Check sheet for the modelled part. Datum: model origin and axes. Units: mm. Face numbers are marked on the shaded views. A direction names the side the tool comes from. Round coordinates to 2 decimals unless told otherwise and drop trailing zeros. Put each result on its own line as item: value. Start each with the question number.
Item 1: Draft check along X on the marked faces 4, 5, 6 and 7. Enter one of: pulls with the +X half, pulls with the -X half, needs draft (parallel to the pull), parting line crosses it, or undercut.
Item 2: Tool access check on the marked faces 1, 2 and 3. Record the directions out of +Z, -Z, +X, -X, +Y, -Y that give a thin tool (end or side, any length) a straight path to the whole face; none if there is none.
Item 3: Section check A-A, the plane z = 2.3. Give the number of separate pieces and of enclosed holes in the cut face, and give its area (3 significant figures).
Item 4: Gauge pin test, flat ends, axial feed: pin 1 Ø4 at (x, y) = (0, 11.11) entering from +Z; pin 2 Ø1 at (x, z) = (4, 1) entering from -Y; pin 3 Ø1 at (x, z) = (9, 1.5) entering from +Y. Record the tip position at first contact, or that the pin passes through.
Item 5: Material ranges on line 1 along Y through (x, z) = (0, 2.05); line 2 along X through (y, z) = (-12.5, 0.8); line 3 along X through (y, z) = (-15, 1.4), recorded low to high.
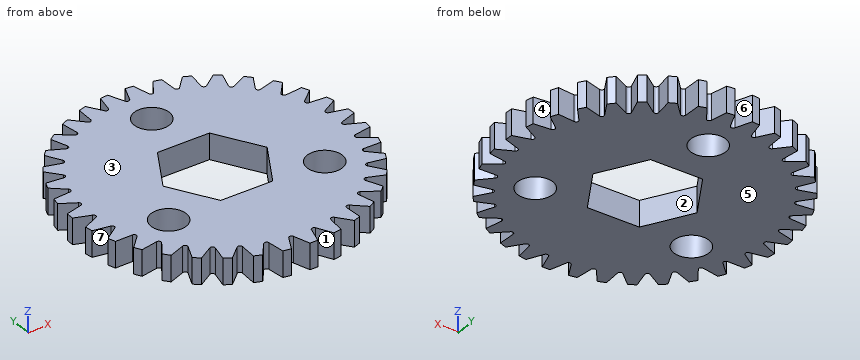
from build123d import *

# Parameters (mm, degrees)
F0_R            = 17.3565013667
F0_R_2          = 2.15265
F1_DEPTH        = 3.175
F3_DEPTH        = 3.175
F3_COPIES_COUNT = 35


# Not quite as in the source:
# - a pattern or mirror of a feature is missing from the dataset's text; its kind, count and spacing are read off the source's solid
# - a feature names something its author has since deleted; it is built from what else it names


with BuildPart() as f1:
    # F0 (on Top) → F1 (new body)
    with BuildSketch(Plane.XY):
        Circle(F0_R)
        with Locations((-9.6237072996, -5.55625)):
            Circle(F0_R_2, mode=Mode.SUBTRACT)
        with Locations((9.6237072996, -5.55625)):
            Circle(F0_R_2, mode=Mode.SUBTRACT)
        Polygon((6.4158048664, 0), (3.2079024332, -5.55625), (-3.2079024332, -5.55625), (-6.4158048664, 0), (-3.2079024332, 5.55625), (3.2079024332, 5.55625), align=None, mode=Mode.SUBTRACT)
        with Locations((0, 11.1125)):
            Circle(F0_R_2, mode=Mode.SUBTRACT)
    extrude(amount=F1_DEPTH)

    # F2 (on face) → F3 (cut, through all)
    with BuildSketch(Plane.XY.offset(3.175)):
        with BuildLine():
            Line((0.275157943, 15.3777549622), (1.0756124971, 17.3231405192))
            ThreePointArc((1.0756124971, 17.3231405192), (0, 17.3565013667), (-1.0756124971, 17.3231405192))
            Line((-1.0756124971, 17.3231405192), (-0.275157943, 15.3777549622))
            ThreePointArc((-0.275157943, 15.3777549622), (0, 15.1934323047), (0.275157943, 15.3777549622))
        make_face()
    f3 = extrude(amount=-F3_DEPTH, mode=Mode.SUBTRACT)

    # F3_copies: F3 ×35 about axis
    f3_copies_axis = Axis((0, 0, 0), (0, 0, 1))
    for i in range(1, F3_COPIES_COUNT):
        add(f3.rotate(f3_copies_axis, i * 360 / F3_COPIES_COUNT), mode=Mode.SUBTRACT)


solid = f1.part
Check result:
1. face 4: pulls with the +X half
1. face 5: needs draft
1. face 6: undercut
1. face 7: pulls with the -X half
2. face 1: +Z, -Z, -Y
2. face 2: +Z, -Z
2. face 3: +Z, +X, -X, +Y, -Y
3. separate pieces: 1
3. enclosed holes: 4
3. area: 700 mm²
4. pin 1: through
4. pin 2: y = -17
4. pin 3: y = 14.09
5. line 1: -17.36 to -5.56, 5.56 to 8.96, 13.27 to 15.19
5. line 2: -11.67 to -9.62, -8.81 to 8.81, 9.62 to 11.67
5. line 3: -8.73 to -8.33, -6.48 to -4.55, -3.81 to 3.81, 4.55 to 6.48, 8.33 to 8.73
